Verification items for the finished model (mm, model axes). Face numbers are marked on the shaded views. A direction names the side the tool comes from. Coordinates: 2 decimals unless noted, no trailing zeros. Write each loop counter-clockwise with the first axis right and the second up, starting at its lowest first coordinate (ties: lowest second). Pieces come first, ordered by that corner, then holes. Notation, with made-up numbers: (-8, 73.5) -> (-1, 73.5) arc R31 cw to (-1, 107.5) -> close; hole circle Ø5 at (-37.75, -10). An arc over 180 degrees is marked (long way). Write item = value, one per line. Start each with the question number.
(1) Set-up check for the marked faces 1, 2, 3 and 4: record each of +Z, -Z, +X, -X, +Y, -Y from which the full face is reachable in a straight line by a thin tool's end or side.
(2) Section check C-C (z = 31.5). Record the cut outline in (x, y), plus the area to 3 significant figures.
(3) Gauge pin test, flat ends, axial feed: pin 1 Ø1.5 at (y, z) = (2, 17) entering from +X; pin 2 Ø3.5 at (y, z) = (12.5, -8) entering from +X; pin 3 Ø4 at (x, z) = (-27.5, 13.5) entering from +Y; pin 4 Ø10 at (y, z) = (9.5, 19) entering from -X. Record the tip position at first contact, or that the pin passes through.
(4) Section check D-D (x = -36.5). Record the cut outline in (y, z).
(5) Material ranges on probe 1 along Z at (x, y) = (-24, 25.5); probe 2 along X at (y, z) = (14.75, 25); probe 3 along Z at (x, y) = (-25.5, 21.25), recorded low to high. Write a range as [from, to].
(6) Section check B-B (y = 20.75). Record the cut outline in (x, z), plus the area to 3 significant figures.
(7) Mould release check, pull along Z, two halves, no side actions. Record for the marked faces 5, 6, 7 and 8: released by +Z, released by -Z, zero draft, split by the parting line, or undercut.
(8) Section check A-A (z = 43). Record the cut outline in (x, y), plus the area to 3 significant figures.
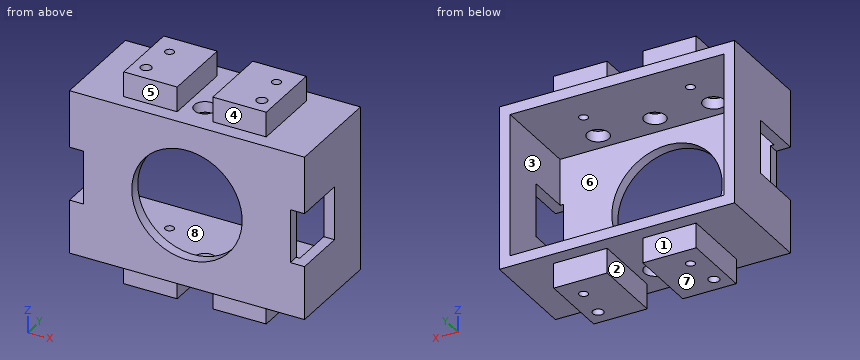
```python
from build123d import *

# Parameters (mm, degrees)
SKETCH1_W               = 66
SKETCH1_H               = 46
BOSS_EXTRUDE2_DEPTH     = 3
SKETCH3_W               = 66
SKETCH3_H               = 46
SKETCH3_W_2             = 60
SKETCH3_H_2             = 40
BOSS_EXTRUDE4_DEPTH     = 25
SKETCH4_W               = 15
SKETCH4_H               = 20
BOSS_EXTRUDE5_DEPTH     = 7
CUT_EXTRUDE1_REACH      = 55
SKETCH5_R               = 1.5
SKETCH5_R_2             = 1.25
SKETCH6_W               = 15
SKETCH6_H               = 20
BOSS_EXTRUDE6_DEPTH     = 7
SKETCH7_R               = 1.5
SKETCH7_R_2             = 1.25
CUT_EXTRUDE2_DEPTH      = 10
CUT_EXTRUDE3_REACH      = 30
SKETCH8_R               = 15.5
SKETCH11_R              = 3
CUT_EXTRUDE6_DEPTH      = 8
CUT_EXTRUDE6_DEPTH_BACK = 54
SKETCH12_R              = 3.025
CUT_EXTRUDE7_DEPTH      = 3
SKETCH14_R              = 3.025
CUT_EXTRUDE8_DEPTH      = 3
SKETCH15_W              = 4
SKETCH15_H              = 15
CUT_EXTRUDE10_DEPTH     = 15


with BuildPart() as part:
    # Sketch1 → Boss-Extrude2 (new body)
    with BuildSketch(Plane(origin=(0, 0, 0), x_dir=(1, 0, 0), z_dir=(0, 1, 0))):
        with Locations((-8.324615879, -17.817795916)):
            Rectangle(SKETCH1_W, SKETCH1_H)
    extrude(amount=BOSS_EXTRUDE2_DEPTH)

    # Sketch3 → Boss-Extrude4 (add)
    with BuildSketch(Plane(origin=(0, 3, 0), x_dir=(1, 0, 0), z_dir=(0, 1, 0))):
        with Locations((-8.324615879, -17.817795916)):
            Rectangle(SKETCH3_W, SKETCH3_H)
        with Locations((-8.324615879, -17.817795916)):
            Rectangle(SKETCH3_W_2, SKETCH3_H_2, mode=Mode.SUBTRACT)
    extrude(amount=BOSS_EXTRUDE4_DEPTH)

    # Sketch4 → Boss-Extrude5 (add)
    with BuildSketch(Plane.XY.offset(40.817795916)):
        with Locations((4.175384121, 14)):
            Rectangle(SKETCH4_W, SKETCH4_H)
        with Locations((-20.824615879, 14)):
            Rectangle(SKETCH4_W, SKETCH4_H)
    extrude(amount=BOSS_EXTRUDE5_DEPTH)

    # Sketch5 → Cut-Extrude1 (cut, up to next)
    with BuildSketch(Plane.XY.offset(47.817795916), mode=Mode.PRIVATE) as cut_extrude1_sk1:
        with Locations((-24.574615879, 8.5)):
            Circle(SKETCH5_R)
    cut_extrude1_tool1 = extrude(cut_extrude1_sk1.sketch, amount=-CUT_EXTRUDE1_REACH, mode=Mode.PRIVATE) & part.part
    add(cut_extrude1_tool1.solids().sort_by_distance((-24.574616, 8.5, 47.817796))[0], mode=Mode.SUBTRACT)
    # Sketch5 → Cut-Extrude1 (cut, up to next)
    with BuildSketch(Plane.XY.offset(47.817795916), mode=Mode.PRIVATE) as cut_extrude1_sk2:
        with Locations((7.925384121, 8.5)):
            Circle(SKETCH5_R)
    cut_extrude1_tool2 = extrude(cut_extrude1_sk2.sketch, amount=-CUT_EXTRUDE1_REACH, mode=Mode.PRIVATE) & part.part
    add(cut_extrude1_tool2.solids().sort_by_distance((7.925384, 8.5, 47.817796))[0], mode=Mode.SUBTRACT)
    # Sketch5 → Cut-Extrude1 (cut, up to next)
    with BuildSketch(Plane.XY.offset(47.817795916), mode=Mode.PRIVATE) as cut_extrude1_sk3:
        with Locations((6.675384121, 18)):
            Circle(SKETCH5_R_2)
    cut_extrude1_tool3 = extrude(cut_extrude1_sk3.sketch, amount=-CUT_EXTRUDE1_REACH, mode=Mode.PRIVATE) & part.part
    add(cut_extrude1_tool3.solids().sort_by_distance((6.675384, 18, 47.817796))[0], mode=Mode.SUBTRACT)
    # Sketch5 → Cut-Extrude1 (cut, up to next)
    with BuildSketch(Plane.XY.offset(47.817795916), mode=Mode.PRIVATE) as cut_extrude1_sk4:
        with Locations((-23.324615879, 18)):
            Circle(SKETCH5_R_2)
    cut_extrude1_tool4 = extrude(cut_extrude1_sk4.sketch, amount=-CUT_EXTRUDE1_REACH, mode=Mode.PRIVATE) & part.part
    add(cut_extrude1_tool4.solids().sort_by_distance((-23.324616, 18, 47.817796))[0], mode=Mode.SUBTRACT)

    # Sketch6 → Boss-Extrude6 (add)
    with BuildSketch(Plane(origin=(0, 0, -5.182204084), x_dir=(-1, 0, 0), z_dir=(0, 0, -1))):
        with Locations((-4.175384121, 14)):
            Rectangle(SKETCH6_W, SKETCH6_H)
        with Locations((20.824615879, 14)):
            Rectangle(SKETCH6_W, SKETCH6_H)
    extrude(amount=BOSS_EXTRUDE6_DEPTH)

    # Sketch7 → Cut-Extrude2 (cut)
    with BuildSketch(Plane(origin=(0, 0, -12.182204084), x_dir=(-1, 0, 0), z_dir=(0, 0, -1))):
        with Locations((-7.925384121, 8.5)):
            Circle(SKETCH7_R)
        with Locations((24.574615879, 8.5)):
            Circle(SKETCH7_R)
        with Locations((23.324615879, 18)):
            Circle(SKETCH7_R_2)
        with Locations((-6.675384121, 18)):
            Circle(SKETCH7_R_2)
    extrude(amount=-CUT_EXTRUDE2_DEPTH, mode=Mode.SUBTRACT)

    # Sketch8 → Cut-Extrude3 (cut, up to next)
    with BuildSketch(Plane(origin=(0, 0, 0), x_dir=(-1, 0, 0), z_dir=(0, -1, 0)), mode=Mode.PRIVATE) as cut_extrude3_sk1:
        with Locations((8.324615879, -17.817795916)):
            Circle(SKETCH8_R)
    cut_extrude3_tool1 = extrude(cut_extrude3_sk1.sketch, amount=-CUT_EXTRUDE3_REACH, mode=Mode.PRIVATE) & part.part
    add(cut_extrude3_tool1.solids().sort_by_distance((-8.324616, 0, 17.817796))[0], mode=Mode.SUBTRACT)

    # Sketch11 → Cut-Extrude6 (cut, two sides)
    with BuildSketch(Plane.XY.offset(40.817795916)) as cut_extrude6_sk:
        with Locations((-8.324615879, 9)):
            Circle(SKETCH11_R)
    extrude(amount=CUT_EXTRUDE6_DEPTH, mode=Mode.SUBTRACT)
    extrude(cut_extrude6_sk.sketch, amount=-CUT_EXTRUDE6_DEPTH_BACK, mode=Mode.SUBTRACT)

    # Sketch12 → Cut-Extrude7 (cut)
    with BuildSketch(Plane(origin=(0, 0, 37.817795916), x_dir=(-1, 0, 0), z_dir=(0, 0, -1))):
        with Locations((24.574615879, 8.5)):
            Circle(SKETCH12_R)
        with Locations((-7.925384121, 8.5)):
            Circle(SKETCH12_R)
    extrude(amount=-CUT_EXTRUDE7_DEPTH, mode=Mode.SUBTRACT)

    # Sketch14 → Cut-Extrude8 (cut)
    with BuildSketch(Plane.XY.offset(-2.182204084)):
        with Locations((-24.574615879, 8.5)):
            Circle(SKETCH14_R)
        with Locations((7.925384121, 8.5)):
            Circle(SKETCH14_R)
    extrude(amount=-CUT_EXTRUDE8_DEPTH, mode=Mode.SUBTRACT)

    # Sketch15 → Cut-Extrude10 (cut)
    with BuildSketch(Plane(origin=(0, 0, 0), x_dir=(-1, 0, 0), z_dir=(0, -1, 0))):
        with Locations((-22.675384121, -17.317795916)):
            Rectangle(SKETCH15_W, SKETCH15_H)
        with Locations((39.324615879, -17.317795916)):
            Rectangle(SKETCH15_W, SKETCH15_H)
    extrude(amount=-CUT_EXTRUDE10_DEPTH, mode=Mode.SUBTRACT)


solid = part.part
```
Response:
q1.face_1 = -Z, +X, -X, +Y
q1.face_2 = -Z, +Y, -Y
q1.face_3 = +Y
q1.face_4 = +Z, +X, -X, -Y
q2.outline = (-41.32, 0) -> (-15.61, 0) -> (-15.61, 3) -> (-38.32, 3) -> (-38.32, 28) -> (-41.32, 28) -> close; (-1.04, 0) -> (24.68, 0) -> (24.68, 28) -> (21.68, 28) -> (21.68, 3) -> (-1.04, 3) -> close
q2.area = 304 mm2
q3.pin_1 = 20.68
q3.pin_2 = 11.68
q3.pin_3 = 3
q3.pin_4 = through
q4.outline = (0, -5.18) -> (28, -5.18) -> (28, -2.18) -> (3, -2.18) -> (3, 37.82) -> (28, 37.82) -> (28, 40.82) -> (0, 40.82) -> close
q5.probe_1 = [-5.18, -2.18], [37.82, 40.82]
q5.probe_2 = [-41.32, -38.32], [21.68, 24.68]
q5.probe_3 = [-12.18, -2.18], [37.82, 47.82]
q6.outline = (-41.32, -5.18) -> (-28.32, -5.18) -> (-28.32, -12.18) -> (-13.32, -12.18) -> (-13.32, -5.18) -> (-3.32, -5.18) -> (-3.32, -12.18) -> (11.68, -12.18) -> (11.68, -5.18) -> (24.68, -5.18) -> (24.68, 40.82) -> (11.68, 40.82) -> (11.68, 47.82) -> (-3.32, 47.82) -> (-3.32, 40.82) -> (-13.32, 40.82) -> (-13.32, 47.82) -> (-28.32, 47.82) -> (-28.32, 40.82) -> (-41.32, 40.82) -> close; hole (-38.32, -2.18) -> (21.68, -2.18) -> (21.68, 37.82) -> (-38.32, 37.82) -> close
q6.area = 1,060 mm2
q7.face_5 = zero draft
q7.face_6 = undercut
q7.face_7 = released by -Z
q7.face_8 = undercut
q8.outline = (-28.32, 4) -> (-13.32, 4) -> (-13.32, 24) -> (-28.32, 24) -> close; (-3.32, 4) -> (11.68, 4) -> (11.68, 24) -> (-3.32, 24) -> close; hole circle Ø3 at (-24.57, 8.5); hole circle Ø2.5 at (-23.32, 18); hole circle Ø2.5 at (6.68, 18); hole circle Ø3 at (7.93, 8.5)
q8.area = 576 mm2
